Here's how the part is built. I have some questions about the finished solid (model axes, mm). Give positions to 0.01 mm unless a question says otherwise; leave off trailing zeros. Write each loop counter-clockwise with the first axis right and the second up, starting at its lowest first coordinate (ties: lowest second). Pieces come first, ordered by that corner, then holes. Notation, with made-up numbers: (-23.75, 74.5) -> (6.25, 74.5) arc R23 cw to (6.25, 109.5) -> close; hole circle Ø3 at (-31.75, 49.25). An arc over 180 degrees is marked (long way). Use one line per item in the form item = value.
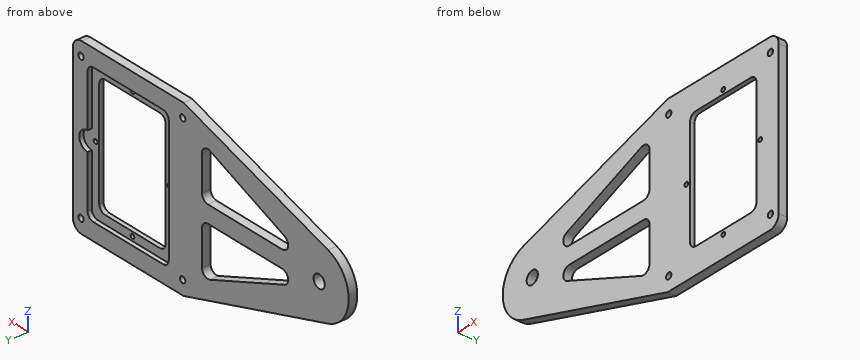
```python
from build123d import *

# Parameters (mm, degrees)
SKETCH1_W           = 95.25
SKETCH1_H           = 127
BOSS_EXTRUDE1_DEPTH = 6.35
BOSS_EXTRUDE3_DEPTH = 6.35
SKETCH5_R           = 4.826
CUT_EXTRUDE1_DEPTH  = 7.35
CUT_EXTRUDE2_DEPTH  = 7.35
FILLET9_R           = 5
SKETCH7_R           = 5.453804141
BOSS_EXTRUDE4_DEPTH = 6.35
SKETCH8_W           = 69.85
SKETCH8_H           = 101.6
CUT_EXTRUDE3_DEPTH  = 3.175
SKETCH9_W           = 57.15
SKETCH9_H           = 88.9
CUT_EXTRUDE4_DEPTH  = 4.175
SKETCH11_R          = 1.5875
CUT_EXTRUDE6_DEPTH  = 4.175
CUT_EXTRUDE7_DEPTH  = 3.175
FILLET10_R          = 5
FILLET11_R          = 5
FILLET12_R          = 7.62
SKETCH13_R          = 2.2812375
CUT_EXTRUDE8_DEPTH  = 7.35


with BuildPart() as part:
    # Sketch1 → Boss-Extrude1 (new body)
    with BuildSketch(Plane(origin=(0, 0, 0), x_dir=(1, 0, 0), z_dir=(0, 1, 0))):
        Rectangle(SKETCH1_W, SKETCH1_H)
    extrude(amount=BOSS_EXTRUDE1_DEPTH)

    # Sketch4 → Boss-Extrude3 (add)
    with BuildSketch(Plane(origin=(0, 6.35, 0), x_dir=(1, 0, 0), z_dir=(0, 1, 0))):
        with BuildLine():
            Line((-47.625, 63.5), (-171.916018217, 24.219268021))
            ThreePointArc((-171.916018217, 24.219268021), (-189.6618, 0), (-171.916018217, -24.219268021))
            Line((-171.916018217, -24.219268021), (-47.625, -63.5))
            Line((-47.625, -63.5), (-47.625, 63.5))
        make_face()
    extrude(amount=-BOSS_EXTRUDE3_DEPTH)

    # Sketch5 → Cut-Extrude1 (cut, through all)
    with BuildSketch(Plane(origin=(0, 6.35, 0), x_dir=(1, 0, 0), z_dir=(0, 1, 0))):
        with Locations((-164.2618, 0)):
            Circle(SKETCH5_R)
        with Locations((-8.6868, 0)):
            Circle(SKETCH5_R)
    extrude(amount=-CUT_EXTRUDE1_DEPTH, mode=Mode.SUBTRACT)

    # Sketch6 → Cut-Extrude2 (cut, through all)
    with BuildSketch(Plane(origin=(0, 6.35, 0), x_dir=(1, 0, 0), z_dir=(0, 1, 0))):
        Polygon((-63.5, 45.163743355), (-157.9118, 6.35), (-63.5, 6.35), align=None)
        Polygon((-63.5, -6.35), (-63.5, -45.163743355), (-157.9118, -6.35), align=None)
    extrude(amount=-CUT_EXTRUDE2_DEPTH, mode=Mode.SUBTRACT)

    # Fillet9
    fillet9_edges = [part.edges().sort_by_distance(p)[0] for p in [
        (-63.5, 3.175, -45.163743355),
        (-63.5, 3.175, -6.35),
        (-157.9118, 3.175, -6.35),
        (-157.9118, 3.175, 6.35),
        (-63.5, 3.175, 6.35),
        (-63.5, 3.175, 45.163743355),
    ]]
    fillet(fillet9_edges, radius=FILLET9_R)

    # Sketch7 → Boss-Extrude4 (add)
    with BuildSketch(Plane(origin=(0, 6.35, 0), x_dir=(1, 0, 0), z_dir=(0, 1, 0))):
        with Locations((-8.6868, 0)):
            Circle(SKETCH7_R)
    extrude(amount=-BOSS_EXTRUDE4_DEPTH)

    # Sketch8 → Cut-Extrude3 (cut)
    with BuildSketch(Plane(origin=(0, 6.35, 0), x_dir=(1, 0, 0), z_dir=(0, 1, 0))):
        Rectangle(SKETCH8_W, SKETCH8_H)
    extrude(amount=-CUT_EXTRUDE3_DEPTH, mode=Mode.SUBTRACT)

    # Sketch9 → Cut-Extrude4 (cut, through all)
    with BuildSketch(Plane(origin=(0, 3.175, 0), x_dir=(1, 0, 0), z_dir=(0, 1, 0))):
        Rectangle(SKETCH9_W, SKETCH9_H)
    extrude(amount=-CUT_EXTRUDE4_DEPTH, mode=Mode.SUBTRACT)

    # Sketch11 → Cut-Extrude6 (cut, through all)
    with BuildSketch(Plane(origin=(0, 3.175, 0), x_dir=(1, 0, 0), z_dir=(0, 1, 0))):
        with Locations((-31.75, 0)):
            Circle(SKETCH11_R)
        with Locations((31.75, 0)):
            Circle(SKETCH11_R)
        with Locations((0, 47.625)):
            Circle(SKETCH11_R)
        with Locations((0, -47.625)):
            Circle(SKETCH11_R)
    extrude(amount=-CUT_EXTRUDE6_DEPTH, mode=Mode.SUBTRACT)

    # Sketch12 → Cut-Extrude7 (cut)
    with BuildSketch(Plane(origin=(0, 6.35, 0), x_dir=(1, 0, 0), z_dir=(0, 1, 0))):
        with BuildLine():
            Line((34.925, 7.112), (34.925, -7.112))
            ThreePointArc((34.925, -7.112), (42.037, 0), (34.925, 7.112))
        make_face()
    extrude(amount=-CUT_EXTRUDE7_DEPTH, mode=Mode.SUBTRACT)

    # Fillet10
    fillet10_edges = [part.edges().sort_by_distance(p)[0] for p in [
        (-34.925, 4.7625, -50.8),
        (34.925, 4.7625, -50.8),
        (34.925, 4.7625, 50.8),
        (-34.925, 4.7625, 50.8),
    ]]
    fillet(fillet10_edges, radius=FILLET10_R)

    # Fillet11
    fillet11_edges = [part.edges().sort_by_distance(p)[0] for p in [
        (-28.575, 1.5875, 44.45),
        (-28.575, 1.5875, -44.45),
        (28.575, 1.5875, -44.45),
        (28.575, 1.5875, 44.45),
    ]]
    fillet(fillet11_edges, radius=FILLET11_R)

    # Fillet12
    fillet12_edges = [part.edges().sort_by_distance(p)[0] for p in [
        (47.625, 3.175, 63.5),
        (47.625, 3.175, -63.5),
    ]]
    fillet(fillet12_edges, radius=FILLET12_R)

    # Sketch13 → Cut-Extrude8 (cut, through all)
    with BuildSketch(Plane(origin=(0, 6.35, 0), x_dir=(1, 0, 0), z_dir=(0, 1, 0))):
        with Locations((-46.889614099, 53.180131976)):
            Circle(SKETCH13_R)
        with Locations((-46.889614099, -53.200246229)):
            Circle(SKETCH13_R)
        with Locations((40.539614099, -53.220360481)):
            Circle(SKETCH13_R)
        with Locations((40.557033552, 53.190189103)):
            Circle(SKETCH13_R)
    extrude(amount=-CUT_EXTRUDE8_DEPTH, mode=Mode.SUBTRACT)


solid = part.part
```
Q1. I want a section at A-A, the plane x = -4. Write out the boundary of the cut face in (y, z) (3 decimals).
Result set:
outline = (0, -63.5) -> (6.35, -63.5) -> (6.35, -50.8) -> (3.175, -50.8) -> (3.175, -44.45) -> (0, -44.45) -> close; (0, 44.45) -> (3.175, 44.45) -> (3.175, 50.8) -> (6.35, 50.8) -> (6.35, 63.5) -> (0, 63.5) -> close
Q2. If I drill on line 1 along Z through (x, y) = (31.75, 1.75); line 2 along Z through (x, y) = (18, 1.75); line 3 along Z through (x, y) = (-126, 5), over which ranges is the centre line in solid material (lowest first)? Write a range as from..to.
Result set:
line_1 = -63.5..-1.59, 1.59..63.5
line_2 = -63.5..-44.45, 44.45..63.5
line_3 = -38.73..-19.47, -6.35..6.35, 19.47..38.73
Q3. Will these pins go through, and if not, where does the flat tip stop? pin 1 Ø1.6 at (y, z) = (1.5, -14) entering from -X; pin 2 Ø3.5 at (y, z) = (5, -19.5) entering from -X; pin 3 Ø1.9 at (x, y) = (-97.5, 2.5) entering from +Z.
Result set:
pin_1 = -185.96
pin_2 = -182.43
pin_3 = 48.04
Q4. I want a section at C-C, the plane x = -121. Write out the boundary of the cut face in (y, z).
Result set:
outline = (0, -40.31) -> (6.35, -40.31) -> (6.35, -21.52) -> (0, -21.52) -> close; (0, -6.35) -> (6.35, -6.35) -> (6.35, 6.35) -> (0, 6.35) -> close; (0, 21.52) -> (6.35, 21.52) -> (6.35, 40.31) -> (0, 40.31) -> close
Q5. I want a section at B-B, the plane z = -31. Write out the boundary of the cut face in (x, y) (3 decimals), and give its area (3 significant figures).
Result set:
outline = (-150.461, 0) -> (-97.952, 0) -> (-97.952, 6.35) -> (-150.461, 6.35) -> close; (-63.5, 0) -> (-28.575, 0) -> (-28.575, 3.175) -> (-34.925, 3.175) -> (-34.925, 6.35) -> (-63.5, 6.35) -> close; (28.575, 0) -> (47.625, 0) -> (47.625, 6.35) -> (34.925, 6.35) -> (34.925, 3.175) -> (28.575, 3.175) -> close
area = 636 mm2
Q6. I want a section at D-D, the plane y = 5. Count the separate pieces of the cut face and the enclosed holes in it, and give its area (3 significant figures).
Result set:
separate_pieces = 1
enclosed_holes = 8
area = 12,900 mm2
